from build123d import *

# Parameters (mm, degrees)
F1_DEPTH  = 12.7
F5_W      = 7.62
F5_H      = 12.7
F6_DEPTH  = 13.97
F8_DEPTH  = 23.876
F9_R      = 6.34999
F10_R     = 5.08
F12_DEPTH = 18.5489899089
F14_DEPTH = 18.5489899089
F15_R     = 1.27


# Not quite as in the source:
# - a fillet or chamfer is up to 0.001 mm smaller than in the source, because OpenCascade refuses the exact size


with BuildPart() as f1:
    # F0 (on Front) → F1 (new body)
    with BuildSketch(Plane.XZ):
        with BuildLine():
            ThreePointArc((56.3854255581, 0.381), (28.194, 28.194), (0.0025744419, 0.381))
            Line((0.0025744419, 0.381), (10.1640250971, 0.381))
            ThreePointArc((10.1640250971, 0.381), (28.194, 18.034), (46.2239749029, 0.381))
            Line((46.2239749029, 0.381), (56.3854255581, 0.381))
        make_face()
    extrude(amount=F1_DEPTH)

    # F3 (on offset) → F4 (join, up to the next surface of F1)
    with BuildSketch(Plane.XY.offset(34.29)):
        Polygon((28.194, 0), (10.16, 0), (10.16, -12.7), (46.228, -12.7), (46.228, 0), align=None)
    extrude(until=Until.NEXT, dir=(0, 0, -1))

    # F5 (on face) → F6 (join)
    with BuildSketch(Plane.XY.offset(34.29)):
        with Locations((20.066, -6.35)):
            Rectangle(F5_W, F5_H)
        with Locations((36.322, -6.35)):
            Rectangle(F5_W, F5_H)
    extrude(amount=F6_DEPTH)

    # F7 (on face) → F8 (cut, through all)
    with BuildSketch(Plane(origin=(16.256, 0, 0), x_dir=(0, -1, 0), z_dir=(-1, 0, 0))):
        with BuildLine():
            ThreePointArc((9.525, 41.91), (8.5950640303, 44.1550640303), (6.35, 45.085))
            ThreePointArc((6.35, 45.085), (4.1049359697, 39.6649359697), (9.525, 41.91))
        make_face()
    extrude(amount=-F8_DEPTH, mode=Mode.SUBTRACT)

    # F9 (radius 6.35 in the source; OpenCascade refuses exactly that, so slightly less here)
    f9_edges = [f1.edges().sort_by_distance(p)[0] for p in [
        (20.066, -12.7, 48.26),
        (20.066, 0, 48.26),
        (36.322, -12.7, 48.26),
        (36.322, 0, 48.26),
    ]]
    fillet(f9_edges, radius=F9_R)

    # F10
    f10_edges = [f1.edges().sort_by_distance(p)[0] for p in [
        (10.16, -6.35, 34.29),
        (10.16, -6.35, 21.672021),
        (46.228, -6.35, 34.29),
        (46.228, -6.35, 21.672021),
    ]]
    fillet(f10_edges, radius=F10_R)

    # F11 (on face) → F12 (cut, up to face)
    with BuildSketch(Plane(origin=(0, 0, 0.381), x_dir=(1, 0, 0), z_dir=(0, 0, -1))):
        with BuildLine():
            ThreePointArc((52.6572502305, 6.35), (52.2610975074, 7.3063972769), (51.3047002305, 7.70255))
            ThreePointArc((51.3047002305, 7.70255), (50.3483029536, 5.3936027231), (52.6572502305, 6.35))
        make_face()
    extrude(amount=-F12_DEPTH, mode=Mode.SUBTRACT)

    # F13 (on face) → F14 (cut, up to face)
    with BuildSketch(Plane(origin=(0, 0, 0.381), x_dir=(1, 0, 0), z_dir=(0, 0, -1))):
        with BuildLine():
            ThreePointArc((6.4358497695, 6.35), (6.0396970464, 7.3063972769), (5.0832997695, 7.70255))
            ThreePointArc((5.0832997695, 7.70255), (4.1269024926, 5.3936027231), (6.4358497695, 6.35))
        make_face()
    extrude(amount=-F14_DEPTH, mode=Mode.SUBTRACT)

    # F15
    f15_edges = [f1.edges().sort_by_distance(p)[0] for p in [
        (28.194, 0, 18.034),
        (2.316329, 0, 11.191416),
        (2.316329, -12.7, 11.191416),
        (28.194, -12.7, 18.034),
        (54.071671, -12.7, 11.191416),
        (54.071671, 0, 11.191416),
        (28.194, 0, 34.29),
        (28.194, -12.7, 34.29),
    ]]
    fillet(f15_edges, radius=F15_R)


solid = f1.part
Design review of the part built by this model. Coordinates are the model's own, in mm. A direction names the side the tool comes from. Give positions to 0.01 mm unless a question says otherwise; leave off trailing zeros. Loops run counter-clockwise (first coordinate to the right, second up) from the corner with the lowest first, then second, coordinate; pieces in that order, holes last. Notation, with made-up numbers: M 54.5,47.5 L 93.5,47.5 A26 cw 93.5,82.5 Z; hole C -2,-1.75 d2. An arc over 180 degrees is marked long. Write item = value, one per line.
Q1. Insertion check: pin 1 (4.5 mm diameter, centred on x = 28, y = -7, fed in from +Z); pin 2 (2 mm diameter, centred on y = -8.5, z = 40, fed in from +X); pin 3 (6 mm diameter, centred on x = 14, y = -9, fed in from +Z); pin 4 (5 mm diameter, centred on y = -6.35, z = 41.91, fed in from +X). Each pin has a flat end and moves straight along its axis. Give the tip position at first contact, or say it passes through.
Output values:
pin_1 = 34.29
pin_2 = 40.13
pin_3 = 48.22
pin_4 = through
Q2. Draft analysis for pull direction X (two halves, no side actions). For faces 6 (the flat face through (10.16, -6, 27)), 7 (the flat face through (28, -6, 34.29)), 8 (the cylindrical face through (54.133, -6.279, 11.048)), 9 (the cylindrical face through (28.254, -12.318, 33.928)), state which applies: +X half, -X half, draft (parallel to the pull), parting line (faces both ways), or undercut.
Output values:
face_6 = -X half
face_7 = undercut
face_8 = +X half
face_9 = undercut
Q3. To check wall thickness, follow line 1 (Y direction, x = 22.25, z = 41.91) (3 decimals); line 2 (X direction, y = -7.25, z = 46); line 3 (X direction, y = -6.35, z = 9.5). State the ranges of each line that lie inside material, in increasing order. Write a range as [from, to].
Output values:
line_1 = [-12.7, -9.525], [-3.175, 0]
line_2 = [16.26, 23.88], [32.51, 40.13]
line_3 = [1.65, 3.73], [6.44, 12.87], [43.52, 49.95], [52.66, 54.74]
Q4. We need section B-B (z = 10.5). Count the separate pieces of the cut face and the enclosed holes in it, plus the area to 3 significant figures.
Output values:
separate_pieces = 2
enclosed_holes = 2
area = 278 mm^2
Q5. For faces 1 (the cylindrical face through (45.846, -0.362, 26.61)), 2 (the cylindrical face through (15.741, -0.362, 33.908)), 3 (the flat face through (46.228, -6, 27)), 4 (the cylindrical face through (10.522, -12.318, 26.536)), 5 (the cylindrical face through (36.38, -10.89, 46.35)), list the 3-axis set-ups (+Z, -Z, +X, -X, +Y, -Y) from which the entire face can be reached by the end or side of a thin tool; tool diameter is ignored.
Output values:
face_1 = +Z, +X, +Y
face_2 = +Z, -X, +Y
face_3 = +Z, +X, +Y, -Y
face_4 = +Z, -X, -Y
face_5 = +Z, +X, -X, -Y
Q6. We need section A-A (z = 36.5). Give the boundary of the cut face in (x, y), plus the area to 3 significant figures.
Output values:
outline = M 16.26,-12.7 L 23.88,-12.7 L 23.88,0 L 16.26,0 Z; M 32.51,-12.7 L 40.13,-12.7 L 40.13,0 L 32.51,0 Z
area = 194 mm^2
